Build history of the part. All positions in model axes, mm. Face numbers are marked on the shaded views. A direction names the side the tool comes from. Coordinates: 2 decimals unless noted, no trailing zeros. Order: outer loops, then holes, each group sorted by start corner. A loop starts at its lowest first (then second) coordinate and runs counter-clockwise, first axis right, second up. Notation, with made-up numbers: (-7, 11.25) - (31, 11.25) arc R17 cw to (31, 16.25) - close; hole circle Ø4 at (61.25, 7). An arc over 180 degrees is marked (long way). Write each question's results on one line, items separated by ' | '.
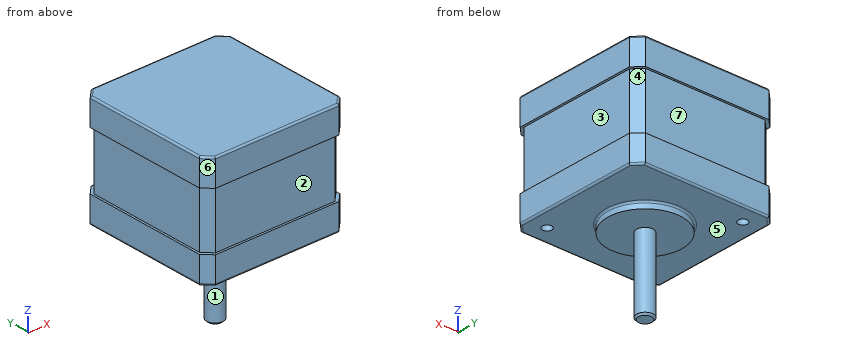
from build123d import *

# Parameters (mm, degrees)
SKETCH1_W           = 41.91
SKETCH1_H           = 41.91
BOSS_EXTRUDE1_DEPTH = 8
SKETCH2_W           = 40.64
SKETCH2_H           = 40.64
BOSS_EXTRUDE2_DEPTH = 17
SKETCH3_W           = 41.91
SKETCH3_H           = 41.91
BOSS_EXTRUDE3_DEPTH = 8
CHAMFER1_SIZE       = 2.54
CHAMFER2_SIZE       = 2.54
SKETCH4_R           = 10.9982
BOSS_EXTRUDE4_DEPTH = 2
SKETCH5_R           = 2.5
BOSS_EXTRUDE5_DEPTH = 22.225
CHAMFER3_SIZE       = 0.508
FILLET2_R           = 0.508
SKETCH6_R           = 1.397
CUT_EXTRUDE1_DEPTH  = 5.08


with BuildPart() as part:
    # Sketch1 → Boss-Extrude1 (new body)
    with BuildSketch(Plane.XY):
        Rectangle(SKETCH1_W, SKETCH1_H)
    extrude(amount=BOSS_EXTRUDE1_DEPTH)

    # Sketch2 → Boss-Extrude2 (add)
    with BuildSketch(Plane.XY.offset(8)):
        Rectangle(SKETCH2_W, SKETCH2_H)
    extrude(amount=BOSS_EXTRUDE2_DEPTH)

    # Sketch3 → Boss-Extrude3 (add)
    with BuildSketch(Plane.XY.offset(25)):
        Rectangle(SKETCH3_W, SKETCH3_H)
    extrude(amount=BOSS_EXTRUDE3_DEPTH)

    # Chamfer1
    chamfer1_edges = [part.edges().sort_by_distance(p)[0] for p in [
        (20.32, -20.32, 16.5),
        (20.32, 20.32, 16.5),
        (-20.32, 20.32, 16.5),
        (-20.32, -20.32, 16.5),
    ]]
    chamfer(chamfer1_edges, length=CHAMFER1_SIZE)

    # Chamfer2
    chamfer2_edges = [part.edges().sort_by_distance(p)[0] for p in [
        (20.955, -20.955, 29),
        (20.955, 20.955, 29),
        (-20.955, 20.955, 29),
        (-20.955, -20.955, 29),
        (20.955, -20.955, 4),
        (-20.955, -20.955, 4),
        (-20.955, 20.955, 4),
        (20.955, 20.955, 4),
    ]]
    chamfer(chamfer2_edges, length=CHAMFER2_SIZE)

    # Sketch4 → Boss-Extrude4 (add)
    with BuildSketch(Plane(origin=(0, 0, 0), x_dir=(-1, 0, 0), z_dir=(0, 0, -1))):
        Circle(SKETCH4_R)
    extrude(amount=BOSS_EXTRUDE4_DEPTH)

    # Sketch5 → Boss-Extrude5 (add)
    with BuildSketch(Plane(origin=(0, 0, -2), x_dir=(-1, 0, 0), z_dir=(0, 0, -1))):
        Circle(SKETCH5_R)
    extrude(amount=BOSS_EXTRUDE5_DEPTH)

    # Chamfer3
    chamfer3_edges = [part.edges().sort_by_distance(p)[0] for p in [
        (2.5, 0, -24.225),
    ]]
    chamfer(chamfer3_edges, length=CHAMFER3_SIZE)

    # Fillet2
    fillet2_edges = [part.edges().sort_by_distance(p)[0] for p in [
        (10.9982, 0, 0),
        (0, 20.955, 33),
        (20.955, 0, 33),
        (-20.955, 0, 33),
        (0, -20.955, 33),
        (19.685, -19.685, 33),
        (-19.685, -19.685, 33),
        (-19.685, 19.685, 33),
        (19.685, 19.685, 33),
        (0, 20.955, 0),
        (20.955, 0, 0),
        (0, -20.955, 0),
        (-20.955, 0, 0),
        (19.685, -19.685, 0),
        (-19.685, -19.685, 0),
        (-19.685, 19.685, 0),
        (19.685, 19.685, 0),
    ]]
    fillet(fillet2_edges, radius=FILLET2_R)

    # Sketch6 → Cut-Extrude1 (cut)
    with BuildSketch(Plane(origin=(0, 0, 0), x_dir=(-1, 0, 0), z_dir=(0, 0, -1))):
        with Locations((15.5, 15.5)):
            Circle(SKETCH6_R)
        with Locations((-15.5, -15.5)):
            Circle(SKETCH6_R)
    extrude(amount=-CUT_EXTRUDE1_DEPTH, mode=Mode.SUBTRACT)


solid = part.part
1. Band-saw the part on A-A on x = -15.5. Give the cut face in (y, z) (3 decimals).
Solved:
outline: (-20.955, 0.508) arc R0.508 ccw to (-20.447, 0) - (14.103, 0) - (14.103, 5.08) - (16.897, 5.08) - (16.897, 0) - (20.447, 0) arc R0.508 ccw to (20.955, 0.508) - (20.955, 8) - (20.32, 8) - (20.32, 25) - (20.955, 25) - (20.955, 32.492) arc R0.508 ccw to (20.447, 33) - (-20.447, 33) arc R0.508 ccw to (-20.955, 32.492) - (-20.955, 25) - (-20.32, 25) - (-20.32, 8) - (-20.955, 8) - close
2. Two-plate mould, pull along Z, no slides. Class the marked faces 4, 5, 6 and 7: +Z half, -Z half, draft (parallel to the pull), parting line (faces both ways), or undercut.
Solved:
face 4: undercut | face 5: -Z half | face 6: draft | face 7: undercut
3. Probe line 1 (Y direction, x = -15.5, z = 3.55) (3 decimals); line 2 (Y direction, x = 15.5, z = 1.35) (3 decimals); line 3 (Z direction, x = -6, y = 4.5). List the from-to ranges inside material, lowest first.
Solved:
line 1: y = -20.955 to 14.103, 16.897 to 20.955 | line 2: y = -20.955 to -16.897, -14.103 to 20.955 | line 3: z = -2 to 33
4. Band-saw the part on C-C on z = -18. Give the cut face in (x, y), then the cut area to 3 significant figures.
Solved:
outline: circle Ø5 at (0, 0) | area: 19.6 mm2
5. Drop flat-ended pins along their axis: pin 1 Ø8 at (x, y) = (-3.5, 15.5) entering from -Z; pin 2 Ø1.5 at (x, z) = (-10.5, 15.5) entering from +Y; pin 3 Ø2 at (y, z) = (-11.5, 20) entering from -X. Give the stop position or say it passes through.
Solved:
pin 1: stops at z = 0 | pin 2: stops at y = 20.32 | pin 3: stops at x = -20.32
6. Band-saw the part on D-D on y = 15.5. Give the cut face in (x, z) (3 decimals), then the cut area to 3 significant figures.
Solved:
outline: (-20.955, 0.508) arc R0.508 ccw to (-20.447, 0) - (-16.897, 0) - (-16.897, 5.08) - (-14.103, 5.08) - (-14.103, 0) - (20.447, 0) arc R0.508 ccw to (20.955, 0.508) - (20.955, 8) - (20.32, 8) - (20.32, 25) - (20.955, 25) - (20.955, 32.492) arc R0.508 ccw to (20.447, 33) - (-20.447, 33) arc R0.508 ccw to (-20.955, 32.492) - (-20.955, 25) - (-20.32, 25) - (-20.32, 8) - (-20.955, 8) - close | area: 1,350 mm2
7. Band-saw the part on B-B on y = 0. Give the cut face in (x, z) (3 decimals), then the cut area to 3 significant figures.
Solved:
outline: (-20.955, 0.508) arc R0.508 ccw to (-20.447, 0) - (-11.506, 0) arc R0.508 cw to (-10.998, -0.508) - (-10.998, -2) - (-2.5, -2) - (-2.5, -23.717) - (-1.992, -24.225) - (1.992, -24.225) - (2.5, -23.717) - (2.5, -2) - (10.998, -2) - (10.998, -0.508) arc R0.508 cw to (11.506, 0) - (20.447, 0) arc R0.508 ccw to (20.955, 0.508) - (20.955, 8) - (20.32, 8) - (20.32, 25) - (20.955, 25) - (20.955, 32.492) arc R0.508 ccw to (20.447, 33) - (-20.447, 33) arc R0.508 ccw to (-20.955, 32.492) - (-20.955, 25) - (-20.32, 25) - (-20.32, 8) - (-20.955, 8) - close | area: 1,520 mm2
8. Tool access for the marked faces 1, 2 and 3: list every direction of +Z, -Z, +X, -X, +Y, -Y with a clear straight run to the whole face (end or side of a thin tool).
Solved:
face 1: -Z | face 2: +X, -X, -Y | face 3: +X, +Y, -Y
